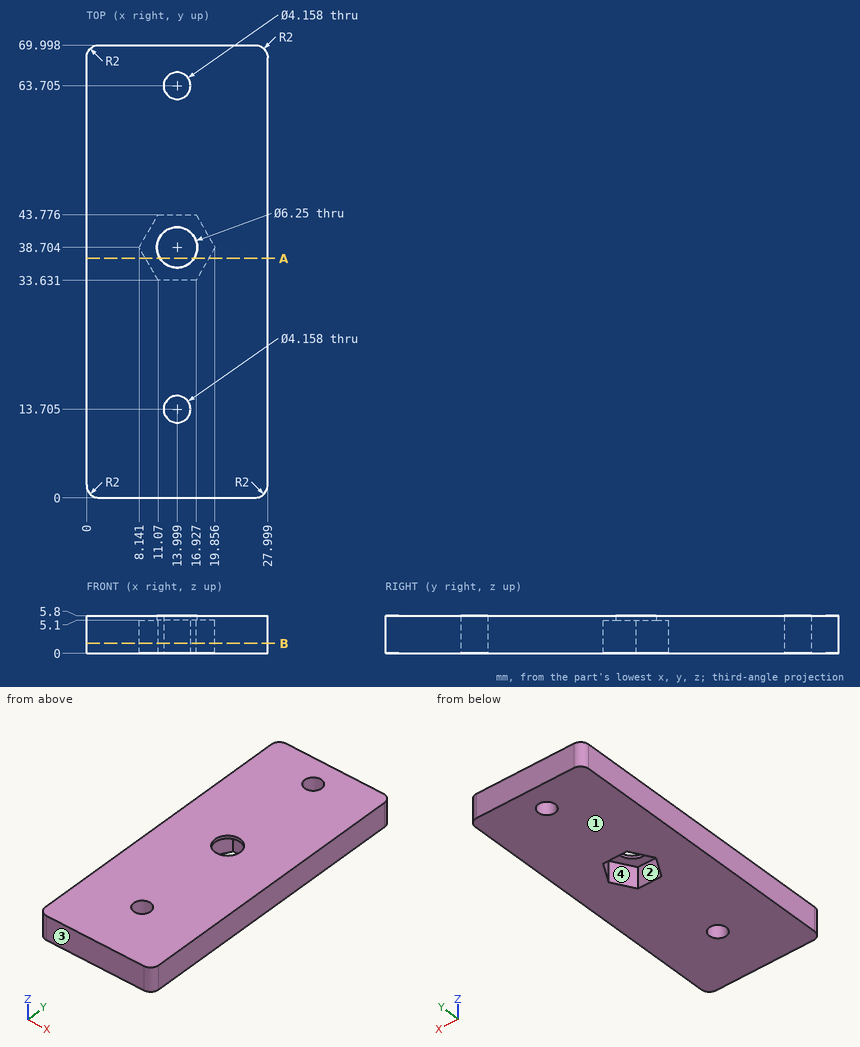
Study the drawing (mm; zero at the part's minimum x, y, z) and answer. Give positions to 0.01 mm unless a question says otherwise; leave off trailing zeros. Write each loop counter-clockwise with the first axis right and the second up, starting at its lowest first coordinate (ties: lowest second). Pieces come first, ordered by that corner, then holes.
(1) The part is cut by section A-A on y = 37. Write down the section's boundary in (x, z) (1 decimal), plus the area to 3 significant figures.
Final values:
outline: (0, 0) - (9.1, 0) - (9.1, 5.1) - (11.4, 5.1) - (11.4, 5.8) - (0, 5.8) - close; (16.6, 5.1) - (18.9, 5.1) - (18.9, 0) - (28, 0) - (28, 5.8) - (16.6, 5.8) - close
area: 109 mm2
(2) A flat-ended cylindrical pin translates along its axis: pin 1 Ø10 at (x, y) = (14, 38.7) entering from -Z. Find the tip coordinate at first contact, or state that the pin passes through.
Final values:
pin 1: stops at z = 5.1
(3) Straight lines are drawn through the part: line 1 (Y direction, x = 12.5, z = 4.8) (1 decimal); line 2 (Y direction, x = 13.5, z = 4.9) (1 decimal); line 3 (Y direction, x = 17.25, z = 2.7) (1 decimal). For each, find the intervals that lie inside material, in ascending order.
Final values:
line 1: y = 0 to 12.3, 15.1 to 33.6, 43.8 to 62.3, 65.1 to 70
line 2: y = 0 to 11.7, 15.7 to 33.6, 43.8 to 61.7, 65.7 to 70
line 3: y = 0 to 34.2, 43.2 to 70
(4) The mould has two halves that part along Y. Classify the marked faces 1, 2, 3 and 4: pulls with the +Y half, pulls with the -Y half, needs draft (parallel to the pull), parting line crosses it, or undercut.
Final values:
face 1: needs draft
face 2: undercut
face 3: pulls with the -Y half
face 4: undercut
(5) The part is cut by section B-B on z = 1.55. Write down the section's boundary in (x, y) (1 decimal), plus the area to 3 significant figures.
Final values:
outline: (0, 2) arc R2 ccw to (2, 0) - (26, 0) arc R2 ccw to (28, 2) - (28, 68) arc R2 ccw to (26, 70) - (2, 70) arc R2 ccw to (0, 68) - close; hole (8.1, 38.7) - (11.1, 33.6) - (16.9, 33.6) - (19.9, 38.7) - (16.9, 43.8) - (11.1, 43.8) - close; hole circle Ø4.2 at (14, 13.7); hole circle Ø4.2 at (14, 63.7)
area: 1,840 mm2
